Source: CAD feature listing. Evaluate the final solid. Frame: model axes, mm. Face numbers are marked on the shaded views. A direction names the side the tool comes from. Round coordinates to 2 decimals unless told otherwise and drop trailing zeros. Loops run counter-clockwise (first coordinate to the right, second up) from the corner with the lowest first, then second, coordinate; pieces in that order, holes last. Notation, with made-up numbers: M -15,69.25 L -6,69.25 A15 cw -6,98.25 Z; hole C 15,53 d10. An arc over 180 degrees is marked long. Answer as CSV lines item,"result". Start each with the question number.
Autodesk Fusion 360 part; units mm, degrees
sketch "Esquisse1" plane through (0, 0, 0) normal (0, 0, 1) x (1, 0, 0)
  circle A0 centre (0, 0) radius 2.25
  line L0 (5.5, -3) -> (25, -3)
  line L1 (25, -3) -> (25, 25) construction
  line L2 (25, 25) -> (-3, 25) construction
  line L3 (-3, 25) -> (-3, 5)
  arc A1 (-3, -1) -> (-1, -3) centre (-1, -1) ccw
  line L4 (-1, 4.5) -> (0, 4.5)
  line L5 (4.5, 0) -> (4.5, -1)
  line L6 (-1, 25) -> (-1, 6.75)
  line L7 (6.76, -1) -> (25, -1)
  arc A2 (4.5, 0) -> (0, 4.5) centre (0, 0) ccw
  line L8 (-0.75, 6.5) -> (0, 6.5)
  line L9 (6.5, 0) -> (6.5, -0.74)
  arc A3 (6.5, 0) -> (0, 6.5) centre (0, 0) ccw
  line L10 (-2.5, 4.5) -> (-1, 4.5)
  line L11 (4.5, -1) -> (4.5, -2)
  arc A4 (6.5, -0.74) -> (6.76, -1) centre (6.76, -0.74) ccw
  arc A5 (-1, 6.75) -> (-0.75, 6.5) centre (-0.75, 6.75) ccw
  arc A6 (4.5, -2) -> (5.5, -3) centre (5.5, -2) ccw
  line L12 (-1, -3) -> (5.5, -3)
  arc A7 (-3, 5) -> (-2.5, 4.5) centre (-2.5, 5) ccw
  line L13 (-3, -1) -> (-3, 5)
  line L14 (45.5, -1) -> (45.5, -2)
  line L15 (53, -1) -> (53, 5)
  line L16 (51, 4.5) -> (50, 4.5)
  line L17 (52.5, 4.5) -> (51, 4.5)
  line L18 (50.75, 6.5) -> (50, 6.5)
  arc A8 (44.5, -3) -> (45.5, -2) centre (44.5, -2) ccw
  arc A9 (50, 4.5) -> (45.5, 0) centre (50, 0) ccw
  line L19 (43.24, -1) -> (25, -1)
  circle A10 centre (50, 0) radius 2.25
  line L20 (51, -3) -> (44.5, -3)
  line L21 (45.5, 0) -> (45.5, -1)
  line L22 (44.5, -3) -> (25, -3)
  arc A11 (52.5, 4.5) -> (53, 5) centre (52.5, 5) ccw
  line L23 (53, 25) -> (53, 5)
  line L24 (51, 25) -> (51, 6.75)
  arc A12 (43.24, -1) -> (43.5, -0.74) centre (43.24, -0.74) ccw
  arc A13 (50.75, 6.5) -> (51, 6.75) centre (50.75, 6.75) ccw
  line L25 (43.5, 0) -> (43.5, -0.74)
  arc A14 (51, -3) -> (53, -1) centre (51, -1) ccw
  arc A15 (50, 6.5) -> (43.5, 0) centre (50, 0) ccw
  line L26 (6.76, 51) -> (25, 51)
  arc A16 (-1, 53) -> (-3, 51) centre (-1, 51) ccw
  line L27 (53, 25) -> (53, 45)
  arc A17 (51, 43.25) -> (50.75, 43.5) centre (50.75, 43.25) ccw
  line L28 (52.5, 45.5) -> (51, 45.5)
  line L29 (45.5, 50) -> (45.5, 51)
  arc A18 (5.5, 53) -> (4.5, 52) centre (5.5, 52) ccw
  line L30 (-1, 53) -> (5.5, 53)
  line L31 (43.24, 51) -> (25, 51)
  arc A19 (53, 51) -> (51, 53) centre (51, 51) ccw
  line L32 (50.75, 43.5) -> (50, 43.5)
  line L33 (5.5, 53) -> (25, 53)
  line L34 (44.5, 53) -> (25, 53)
  line L35 (51, 45.5) -> (50, 45.5)
  arc A20 (-0.75, 43.5) -> (-1, 43.25) centre (-0.75, 43.25) ccw
  arc A21 (0, 45.5) -> (4.5, 50) centre (0, 50) ccw
  line L36 (4.5, 50) -> (4.5, 51)
  line L37 (-1, 25) -> (-1, 43.25)
  line L38 (4.5, 51) -> (4.5, 52)
  line L39 (6.5, 50) -> (6.5, 50.74)
  line L40 (51, 25) -> (51, 43.25)
  line L41 (-1, 45.5) -> (0, 45.5)
  line L42 (51, 53) -> (44.5, 53)
  line L43 (45.5, 51) -> (45.5, 52)
  arc A22 (43.5, 50.74) -> (43.24, 51) centre (43.24, 50.74) ccw
  arc A23 (53, 45) -> (52.5, 45.5) centre (52.5, 45) ccw
  arc A24 (0, 43.5) -> (6.5, 50) centre (0, 50) ccw
  line L44 (53, 51) -> (53, 45)
  arc A25 (6.76, 51) -> (6.5, 50.74) centre (6.76, 50.74) ccw
  line L45 (-3, 25) -> (-3, 45)
  arc A26 (45.5, 52) -> (44.5, 53) centre (44.5, 52) ccw
  arc A27 (43.5, 50) -> (50, 43.5) centre (50, 50) ccw
  circle A28 centre (0, 50) radius 2.25
  line L46 (43.5, 50) -> (43.5, 50.74)
  circle A29 centre (50, 50) radius 2.25
  line L47 (-0.75, 43.5) -> (0, 43.5)
  line L48 (-3, 51) -> (-3, 45)
  arc A30 (45.5, 50) -> (50, 45.5) centre (50, 50) ccw
  arc A31 (-2.5, 45.5) -> (-3, 45) centre (-2.5, 45) ccw
  line L49 (-2.5, 45.5) -> (-1, 45.5)
  circle A32 centre (25, 25) radius 13
  point P0 (50, 0)
  point P1 (25, 25)
  point P2 (25, 25)
  point P3 (25, 25)
  point P4 (0, 50)
  point P5 (50, 50)
  dimension "d22" = 4.5
  dimension "d23" = 3
  dimension "d24" = 3
  dimension "d25" = 2
  dimension "d30" = 25
  dimension "d31" = 25
  dimension "d32" = 2
  dimension "d33" = 2
  dimension "d34" = 4.5
  dimension "d35" = 4.5
  dimension "d36" = 4.5
  dimension "d37" = 2
  dimension "d38" = 2
  dimension "d39" = 6.5
  dimension "d40" = 0.26
  dimension "d41" = 0.25
  dimension "d42" = 1
  dimension "d43" = 0.5
  dimension "d44" = 26
extrude "Extrusion1" add sketch "Esquisse1" along normal blind 4 contours L0 L3 L4 L5 A2 L10 L11 A6 A7 L14 L16 L17 A8 A9 L21 L22 A11 L23 L27 L28 L29 A18 L33 L34 L35 A21 L36 L38 L41 L43 A23 L45 A26 A30 A31 L49 | A1 L4 L5 A2 L10 L11 A6 L12 A7 L13 | L14 L15 L16 L17 A8 A9 L20 L21 A11 A14 | A16 A18 L30 A21 L36 L38 L41 L48 A31 L49 | L28 L29 A19 L35 L42 L43 A23 L44 A26 A30
extrude "Extrusion2" add sketch "Esquisse1" along normal blind 16.9 from surface at 4 contours L0 L3 L4 L5 A2 L10 L11 A6 A7 L14 L16 L17 A8 A9 L21 L22 A11 L23 L27 L28 L29 A18 L33 L34 L35 A21 L36 L38 L41 L43 A23 L45 A26 A30 A31 L49
extrude "Extrusion3" add sketch "Esquisse1" along normal blind 1 from surface at 20.9 contours L0 L3 L4 L5 A2 L10 L11 A6 A7 L14 L16 L17 A8 A9 L21 L22 A11 L23 L27 L28 L29 A18 L33 L34 L35 A21 L36 L38 L41 L43 A23 L45 A26 A30 A31 L49 | L6 L7 L8 L9 A3 A4 A5 L18 L19 L24 A12 A13 L25 A15 L26 A17 L31 L32 A20 L37 L39 L40 A22 A24 A25 A27 L46 L47
equation "d48 = 8.9 mm + 8 mm"
equation "d50 = 12.9 mm + 8 mm"
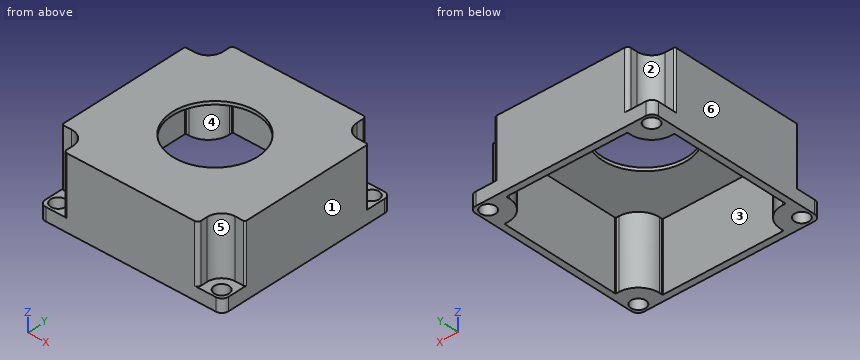
1) Section C-C, the plane x = 10. Return loops of the section in (y, z).
2) Section A-A, the plane x = 25. Return loops of the section in (y, z), and give its area (3 significant figures).
3) Access query for the marked faces 4, 5 and 6. Directions: +Z, -Z, +X, -X, +Y, -Y. A direction counts if a zero-diameter tool reaches every point of the face in a straight line with its end or side. Return the directions, or none.
4) Section D-D, the plane x = 3.5. Return loops of the section in (y, z), and give its area (3 significant figures).
5) Contact query for flat-ended pins moving along their axis: pin 1 Ø6 at (x, y) = (50, 50) entering from +Z; pin 2 Ø9 at (x, y) = (1.5, 2.5) entering from +Z; pin 3 Ø0.8 at (y, z) = (50.5, 6) entering from -X; pin 4 Ø1 at (x, y) = (43, 15.5) entering from -Z. Output: stop coordinate, or through.
6) Mould query, pull axis X, two halves, no side actions, for the marked faces 1, 2 and 3. Classes: pulls with the +X half, pulls with the -X half, needs draft (parallel to the pull), parting line crosses it, or undercut.
7) Ray query, line 1 along Y through (x, z) = (50, 1.8); line 2 along Y through (x, z) = (25, 21.55); line 3 along Y through (x, z) = (22, 19.25). Return the intervals inside material, ascending.
Findings below:
1,outline,"M -3,0 L -1,0 L -1,20.9 L 51,20.9 L 51,0 L 53,0 L 53,21.9 L -3,21.9 Z"
2,outline,"M -3,0 L -1,0 L -1,20.9 L 12,20.9 L 12,21.9 L -3,21.9 Z; M 38,20.9 L 51,20.9 L 51,0 L 53,0 L 53,21.9 L 38,21.9 Z"
2,area,"114 mm²"
3,face 4,"-Z"
3,face 5,"+Z, +X, -Y"
3,face 6,"+Z, -Z, -X, +Y, -Y"
4,outline,"M -3,0 L 5.48,0 L 5.48,20.9 L 44.52,20.9 L 44.52,0 L 53,0 L 53,4 L 47.17,4 L 47.17,21.9 L 2.83,21.9 L 2.83,4 L -3,4 Z"
4,area,"202 mm²"
5,pin 1,"z = 4"
5,pin 2,"z = 21.9"
5,pin 3,"x = 4.5"
5,pin 4,"z = 20.9"
6,face 1,"pulls with the +X half"
6,face 2,"pulls with the -X half"
6,face 3,"undercut"
7,line 1,"-3 to -2.25, 2.25 to 6.5, 43.5 to 47.75, 52.25 to 53"
7,line 2,"-3 to 12, 38 to 53"
7,line 3,"-3 to -1, 51 to 53"
